```python
from build123d import *

# Parameters (mm, degrees)
SKETCH_1_R      = 2.5
EXTRUDE_1_DEPTH = 3.6


with BuildPart() as part:
    # Эскиз1 → Вытянуть1 (new body)
    with BuildSketch(Plane.XY):
        Polygon((0, 4.618802154), (-4, 2.309401077), (-4, -2.309401077), (0, -4.618802154), (4, -2.309401077), (4, 2.309401077), align=None)
        with Locations(Location((0, 0, 0), (0, 0, 180))):
            Circle(SKETCH_1_R, mode=Mode.SUBTRACT)
    extrude(amount=EXTRUDE_1_DEPTH)


solid = part.part
```
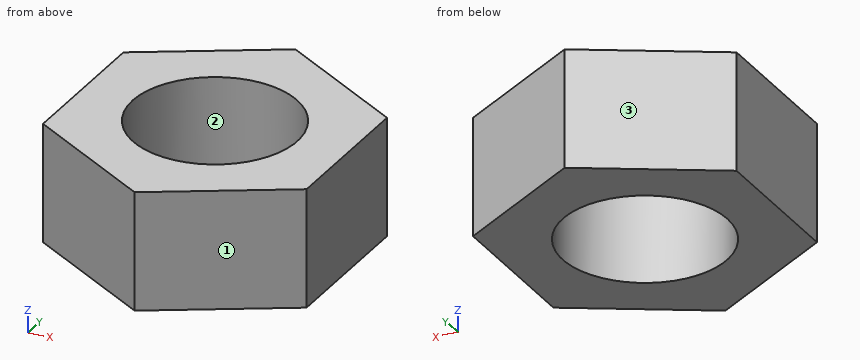
Geometry: final body of the model. Coordinates: model frame, mm. Face numbers are marked on the shaded views. Coordinates: 2 decimals unless noted, no trailing zeros. Write each loop counter-clockwise with the first axis right and the second up, starting at its lowest first coordinate (ties: lowest second). Pieces come first, ordered by that corner, then holes. Notation, with made-up numbers: M 18.5,15.5 L 43.5,15.5 A8 ccw 43.5,26.5 Z; hole C -1,11 d2. An arc over 180 degrees is marked long. Use CSV: the item, a comma, the result in double quotes. Start each with the question number.
1. Ray query, probe 1 along Y at (x, z) = (-0.25, 2.1); probe 2 along Y at (x, z) = (1.5, 3.25); probe 3 along X at (y, z) = (3.5, 2.75). Return the intervals inside material, ascending.
2. First-contact query: P1, Ø1, axis at x = 2.5, z = 1, coming from the -Y side; P2, Ø2, axis at x = 1.5, z = 2, coming from the -Y side. Flat tips, straight axial feed; report the tip coordinate or a pass-through.
3. Cut plane A-A on y = 0. Return the cut outline in (x, z).
4. Cut plane C-C on x = -1.5. Return the cut outline in (y, z).
5. Mould query, pull axis Y, two halves, no side actions, for the marked faces 1, 2 and 3. Classes: pulls with the +Y half, pulls with the -Y half, needs draft (parallel to the pull), parting line crosses it, or undercut.
6. Cut plane B-B on z = 1.05. Return the cut outline in (x, y), plus the area to 3 significant figures.
7. Cut plane D-D on y = 4.25. Return the cut outline in (x, z).
Entries:
1,probe 1,"-4.47 to -2.49, 2.49 to 4.47"
1,probe 2,"-3.75 to -2, 2 to 3.75"
1,probe 3,"-1.94 to 1.94"
2,P1,"y = -3.46"
2,P2,"y = -4.33"
3,outline,"M -4,0 L -2.5,0 L -2.5,3.6 L -4,3.6 Z; M 2.5,0 L 4,0 L 4,3.6 L 2.5,3.6 Z"
4,outline,"M -3.75,0 L -2,0 L -2,3.6 L -3.75,3.6 Z; M 2,0 L 3.75,0 L 3.75,3.6 L 2,3.6 Z"
5,face 1,"pulls with the -Y half"
5,face 2,"undercut"
5,face 3,"pulls with the +Y half"
6,outline,"M -4,-2.31 L 0,-4.62 L 4,-2.31 L 4,2.31 L 0,4.62 L -4,2.31 Z; hole C 0,0 d5"
6,area,"35.8 mm²"
7,outline,"M -0.64,0 L 0.64,0 L 0.64,3.6 L -0.64,3.6 Z"
